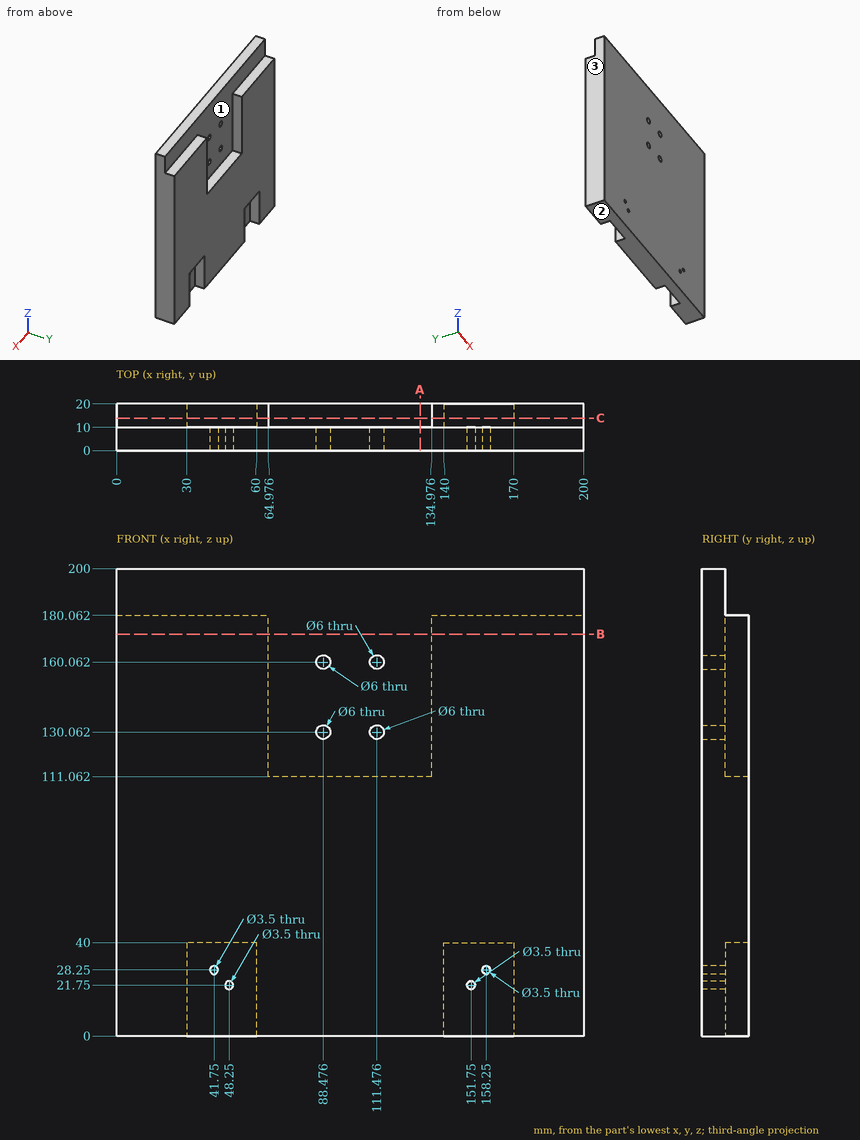
Verification items for this drawing (mm, ordinates from the low corner). Coordinates: 2 decimals unless noted, no trailing zeros. Order: outer loops, then holes, each group sorted by start corner. A loop starts at its lowest first (then second) coordinate and runs counter-clockwise, first axis right, second up. Notation, with made-up numbers: (24.5, 76.25) - (51.5, 76.25) arc R29 ccw to (51.5, 101.25) - close; hole circle Ø7 at (73.25, 73.25). An arc over 180 degrees is marked (long way). Answer as a JSON object with one key per item and string values. Group by question number.
Item 1: Depth check by flat-ended pin: pin 1 Ø3 at (x, y) = (157, 13.5) entering from +Z; pin 2 Ø5 at (x, z) = (111.48, 130.06) entering from +Y. Enter the tip coordinate at first touch or a pass-through.
Item 2: Sectioned sample at A-A, the plane x = 130. Record the cut outline in (y, z), and give its area (3 significant figures).
Item 3: Sectioned sample at B-B, the plane z = 172. Record the cut outline in (x, y).
Item 4: Scan lines: probe 1 along X at (y, z) = (5.75, 28.25); probe 2 along Z at (x, y) = (48.25, 3.5); probe 3 along X at (y, z) = (18.25, 155.5). Record each from-to range of solid material in increasing order.
Item 5: Draft check along X on the marked faces 1, 2 and 3. Enter one of: +X half, -X half, draft (parallel to the pull), parting line (faces both ways), or undercut.
Item 6: Sectioned sample at C-C, the plane y = 14. Record the cut outline in (x, z).
Resolved:
{
 "1": {"pin 1": "z = 180.06", "pin 2": "through"},
 "2": {"outline": "(0, 0) - (20, 0) - (20, 111.06) - (10, 111.06) - (10, 200) - (0, 200) - close", "area": "3,110 mm^2"},
 "3": {"outline": "(0, 0) - (200, 0) - (200, 20) - (134.98, 20) - (134.98, 10) - (64.98, 10) - (64.98, 20) - (0, 20) - close"},
 "4": {"probe 1": "0 to 40, 43.5 to 156.5, 160 to 200", "probe 2": "0 to 20, 23.5 to 200", "probe 3": "0 to 64.98, 134.98 to 200"},
 "5": {"face 1": "undercut", "face 2": "draft", "face 3": "-X half"},
 "6": {"outline": "(0, 0) - (30, 0) - (30, 40) - (60, 40) - (60, 0) - (140, 0) - (140, 40) - (170, 40) - (170, 0) - (200, 0) - (200, 180.06) - (134.98, 180.06) - (134.98, 111.06) - (64.98, 111.06) - (64.98, 180.06) - (0, 180.06) - close"}
}
